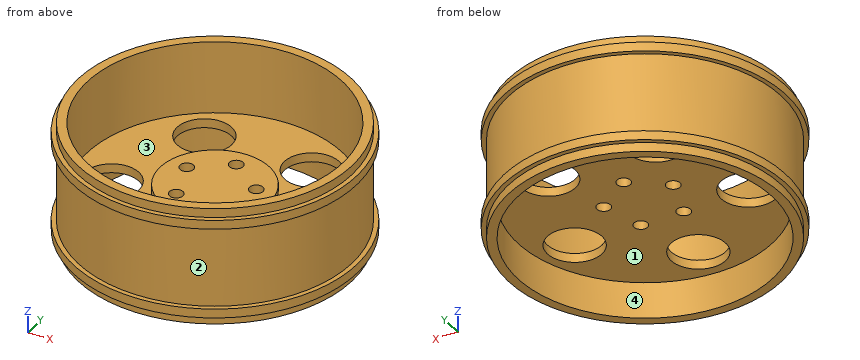
```python
from build123d import *

# Parameters (mm, degrees)
SKETCH8_R               = 7.5
CUT_EXTRUDE1_DEPTH      = 71
CUT_EXTRUDE1_DEPTH_BACK = 61
SKETCH9_R               = 30
CUT_EXTRUDE2_DEPTH      = 81
CUT_EXTRUDE2_DEPTH_BACK = 51


with BuildPart() as part:
    # Sketch6 → Revolve3 (revolve)
    with BuildSketch(Plane(origin=(0, 0, 0), x_dir=(0, 0, -1), z_dir=(1, 0, 0))):
        Polygon((0, 0), (10, 0), (10, 140), (50, 140), (50, 150), (40, 150), (40, 155), (30, 155), (30, 150), (-60, 150), (-60, 155), (-70, 155), (-70, 150), (-80, 150), (-80, 140), (0, 140), (0, 60), (-10, 60), (-10, 0), align=None)
    revolve(axis=Axis((0, 0, 10), (0, 0, -1)))

    # Sketch8 → Cut-Extrude1 (cut, two sides)
    with BuildSketch(Plane.XY.offset(10)) as cut_extrude1_sk:
        with Locations((0, 40)):
            Circle(SKETCH8_R)
        with Locations((38.042260652, 12.360679775)):
            Circle(SKETCH8_R)
        with Locations((23.511410092, -32.360679775)):
            Circle(SKETCH8_R)
        with Locations((-23.511410092, -32.360679775)):
            Circle(SKETCH8_R)
        with Locations((-38.042260652, 12.360679775)):
            Circle(SKETCH8_R)
    extrude(amount=CUT_EXTRUDE1_DEPTH, mode=Mode.SUBTRACT)
    extrude(cut_extrude1_sk.sketch, amount=-CUT_EXTRUDE1_DEPTH_BACK, mode=Mode.SUBTRACT)

    # Sketch9 → Cut-Extrude2 (cut, two sides)
    with BuildSketch(Plane.XY) as cut_extrude2_sk:
        with Locations((0, -100)):
            Circle(SKETCH9_R)
        with Locations((-95.10565163, -30.901699437)):
            Circle(SKETCH9_R)
        with Locations((-58.778525229, 80.901699437)):
            Circle(SKETCH9_R)
        with Locations((58.778525229, 80.901699437)):
            Circle(SKETCH9_R)
        with Locations((95.10565163, -30.901699437)):
            Circle(SKETCH9_R)
    extrude(amount=CUT_EXTRUDE2_DEPTH, mode=Mode.SUBTRACT)
    extrude(cut_extrude2_sk.sketch, amount=-CUT_EXTRUDE2_DEPTH_BACK, mode=Mode.SUBTRACT)


solid = part.part
```
Check sheet for the modelled part. Datum: model origin and axes. Units: mm. Face numbers are marked on the shaded views. A direction names the side the tool comes from. Round coordinates to 2 decimals unless told otherwise and drop trailing zeros. Put each result on its own line as item: value.
(1) Tool access check on the marked faces 3 and 4. Record the directions out of +Z, -Z, +X, -X, +Y, -Y that give a thin tool (end or side, any length) a straight path to the whole face; none if there is none.
Values found:
face 3: +Z
face 4: -Z
(2) Go/stop test with flat-tipped pins: pin 1 Ø1 at (y, z) = (27.5, -26.5) entering from +X; pin 2 Ø6 at (y, z) = (-103, -20) entering from -X; pin 3 Ø19.5 at (x, y) = (38.04, 12.36) entering from -Z. Record where each tip stops, or that it passes through.
Values found:
pin 1: stops at x = 147.55
pin 2: stops at x = -111.8
pin 3: stops at z = -10
(3) Mould release check, pull along Y, two halves, no side actions. Record for the marked faces 1 and 2: released by +Y, released by -Y, zero draft, split by the parting line, or undercut.
Values found:
face 1: undercut
face 2: split by the parting line
(4) Sectioned sample at B-B (z = -5). Count the separate pieces of the cut face and the enclosed holes in it, plus the area to 3 significant figures.
Values found:
separate pieces: 1
enclosed holes: 10
area: 55,700 mm^2
(5) Material ranges on line 1 (Y direction, x = 26.5, z = 6); line 2 (Y direction, x = -2.5, z = -39); line 3 (X direction, y = -23, z = -4), recorded low to high.
Values found:
line 1: y = -147.64 to -137.47, -53.83 to -39.24, -25.48 to 53.83, 137.47 to 147.64
line 2: y = -154.98 to -139.98, 139.98 to 154.98
line 3: x = -148.23 to -124.05, -66.16 to 66.16, 124.05 to 148.23
